Part model, mm, in its own coordinate system. A direction names the side the tool comes from. Round coordinates to 2 decimals unless told otherwise and drop trailing zeros. Write each loop counter-clockwise with the first axis right and the second up, starting at its lowest first coordinate (ties: lowest second). Pieces come first, ordered by that corner, then holes.
1) Saw through at A-A on y = -39.76. Write the cut outline in (x, z), and give its area (3 significant figures).
2) Which spindle directions (+Z, -Z, +X, -X, +Y, -Y) get a long thin tool onto all of the face, cutting with end or side? Do faces 1 (the flat face through (4, -15, 20)), 2 (the flat face through (4, 35.76, -16)), 3 (the cylindrical face through (2, 52, 0)). Say none if no direction does.
3) Saw through at D-D on z = -18.5. Write the cut outline in (x, y), and give its area (3 significant figures).
4) Saw through at C-C on y = 41.76. Write the cut outline in (x, z) (3 decimals).
5) Flat gauge pins, fed straight in: pin 1 (2.5 mm diameter, centred on x = 7, y = 51.5, fed in from +Z); pin 2 (1.5 mm diameter, centred on x = 5.5, y = 6.5, fed in from -Z); pin 3 (2.5 mm diameter, centred on x = 6.5, y = 52, fed in from -Z); pin 4 (5.5 mm diameter, centred on y = -39.76, z = 17, fed in from -X). Where does each tip first touch, or does it go through?
6) Drill centre lines: L1, parallel to Y at x = 2.5, z = 16; L2, parallel to Y at x = 4, z = 17; L3, parallel to Z at x = 4, y = 48. Where is each one in solid material? Low to high.
7) Pull direction Y, two halves, no side cores. Call faces 4 (the flat face through (7, 52, 1.25)), 5 (the flat face through (4, -47.76, 17)), 6 (the cylindrical face through (3.94, 38.83, 16.35)): +Y half, -Y half, draft (parallel to the pull), parting line (faces both ways), or undercut.
8) Saw through at B-B on x = 4. Count the separate pieces of the cut face and the enclosed holes in it, and give its area (3 significant figures).
```python
from build123d import *

# Parameters (mm, degrees)
SKETCH1_W                       = 46
SKETCH1_H                       = 95.52
BOSS_EXTRUDE1_DEPTH             = 8
F_6_0MM_CLEARANCE_DOWEL_HOLE1_D = 6
SKETCH4_W                       = 8
SKETCH4_H                       = 46
BOSS_EXTRUDE2_DEPTH             = 12
FILLET1_R                       = 10
SKETCH6_R                       = 2
CUT_EXTRUDE2_DEPTH              = 15
SKETCH9_W                       = 26
SKETCH9_H                       = 30.52
CUT_EXTRUDE5_DEPTH              = 65.531059189
F_6_0MM_CLEARANCE_DOWEL_HOLE2_D = 6
CUT_EXTRUDE13_DEPTH             = 65.531059189
SKETCH7_W                       = 2.5
SKETCH7_H                       = 15
CUT_EXTRUDE12_DEPTH             = 4
SKETCH16_W                      = 34
SKETCH16_H                      = 53
CUT_EXTRUDE9_DEPTH              = 65.531059294
CUT_EXTRUDE14_DEPTH             = 65.531059294
CUT_EXTRUDE15_DEPTH             = 65.531059294
FILLET2_START                   = -1
FILLET2_DEPTH                   = 10
SKETCH22_R                      = 3
CUT_EXTRUDE16_DEPTH             = 65.531059329


with BuildPart() as part:
    # Sketch1 → Boss-Extrude1 (new body)
    with BuildSketch(Plane(origin=(0, 0, 0), x_dir=(0, 0, -1), z_dir=(1, 0, 0))):
        Rectangle(SKETCH1_W, SKETCH1_H)
    extrude(amount=BOSS_EXTRUDE1_DEPTH)

    # Ø6.0mm Clearance Dowel Hole1 (through all)
    with Locations(Plane(origin=(8, 0, 0), x_dir=(0, 0, -1), z_dir=(1, 0, 0))):
        with Locations((-17, 41.76), (17, 41.76)):
            Hole(F_6_0MM_CLEARANCE_DOWEL_HOLE1_D / 2)

    # Sketch4 → Boss-Extrude2 (add)
    with BuildSketch(Plane(origin=(0, 47.76, 0), x_dir=(1, 0, 0), z_dir=(0, 1, 0))):
        with Locations((4, 0)):
            Rectangle(SKETCH4_W, SKETCH4_H)
    extrude(amount=BOSS_EXTRUDE2_DEPTH)

    # Fillet1
    fillet1_edges = [part.edges().sort_by_distance(p)[0] for p in [
        (4, 59.76, 23),
        (4, 59.76, -23),
    ]]
    fillet(fillet1_edges, radius=FILLET1_R)

    # Sketch6 → Cut-Extrude2 (cut)
    with BuildSketch(Plane(origin=(0, 59.76, 0), x_dir=(1, 0, 0), z_dir=(0, 1, 0))):
        with Locations(Location((4, 0, 0), (0, 0, 270))):
            Circle(SKETCH6_R)
    extrude(amount=-CUT_EXTRUDE2_DEPTH, mode=Mode.SUBTRACT)

    # Sketch9 → Cut-Extrude5 (cut, through all)
    with BuildSketch(Plane(origin=(8, 0, 0), x_dir=(0, 0, -1), z_dir=(1, 0, 0))):
        with Locations((10, 20.5)):
            Rectangle(SKETCH9_W, SKETCH9_H)
    extrude(amount=-CUT_EXTRUDE5_DEPTH, mode=Mode.SUBTRACT)

    # Ø6.0mm Clearance Dowel Hole2 (through all)
    with Locations(Plane(origin=(8, 0, 0), x_dir=(0, 0, -1), z_dir=(1, 0, 0))):
        with Locations((-17, -39.76)):
            Hole(F_6_0MM_CLEARANCE_DOWEL_HOLE2_D / 2)

    # Sketch14 → Cut-Extrude13 (cut, through all)
    with BuildSketch(Plane(origin=(8, 0, 0), x_dir=(0, 0, -1), z_dir=(1, 0, 0))):
        with BuildLine():
            Line((5, 40.013359235), (5, 35.76))
            Line((5, 35.76), (-5, 35.76))
            Line((-5, 35.76), (-5, 40.013359235))
            ThreePointArc((-5, 40.013359235), (0, 45.013359235), (5, 40.013359235))
        make_face()
    extrude(amount=-CUT_EXTRUDE13_DEPTH, mode=Mode.SUBTRACT)

    # Sketch7 → Cut-Extrude12 (cut)
    with BuildSketch(Plane(origin=(8, 0, 0), x_dir=(0, 0, -1), z_dir=(1, 0, 0))):
        with Locations((0, 52.26)):
            Rectangle(SKETCH7_W, SKETCH7_H)
    extrude(amount=-CUT_EXTRUDE12_DEPTH, mode=Mode.SUBTRACT)

    # Sketch16 → Cut-Extrude9 (cut, through all)
    with BuildSketch(Plane(origin=(8, 0, 0), x_dir=(0, 0, -1), z_dir=(1, 0, 0))):
        with Locations((6, -21.26)):
            Rectangle(SKETCH16_W, SKETCH16_H)
    extrude(amount=-CUT_EXTRUDE9_DEPTH, mode=Mode.SUBTRACT)

    # Sketch19 → Cut-Extrude14 (cut, through all)
    with BuildSketch(Plane(origin=(8, 0, 0), x_dir=(0, 0, -1), z_dir=(1, 0, 0))):
        Polygon((-5, 35.76), (3.485281374, 27.274718626), (10.556349186, 34.345786438), (2.071067812, 42.831067812), align=None)
    extrude(amount=-CUT_EXTRUDE14_DEPTH, mode=Mode.SUBTRACT)

    # Sketch21 → Cut-Extrude15 (cut, through all)
    with BuildSketch(Plane(origin=(8, 0, 0), x_dir=(0, 0, -1), z_dir=(1, 0, 0))):
        Polygon((-3, 7.538097039), (-5.298097039, 5.24), (-3, 5.24), align=None)
    extrude(amount=-CUT_EXTRUDE15_DEPTH, mode=Mode.SUBTRACT)

    # Fillet2: read off the stored shape, not the designer's step
    # Fillet2 outline → Fillet2 (cut)
    with BuildSketch(Plane.YZ.offset(FILLET2_START)):
        with BuildLine():
            add(Edge.make_bspline(
                [(40.779548187, -4.94094672), (39.810996275, -5.091139348), (39.117941215, -5.784194408)],
                knots=[0, 0, 0, 1, 1, 1], degree=2))
            ThreePointArc((40.779548187, -4.94094672), (40.397589895, -4.98521482), (40.013359235, -5))
            Line((40.013359235, -5), (39.902135624, -5))
            Line((39.902135624, -5), (39.117941215, -5.784194408))
        make_face()
    extrude(amount=FILLET2_DEPTH, mode=Mode.SUBTRACT)

    # Fillet3
    # a fillet whose section is not a circle: 3 mm, written as the material it adds along each edge
    with BuildSketch(Plane(origin=(8, 35.76, 5), x_dir=(0, 1, 0), z_dir=(-1, 0, 0))) as fillet3_piece_1:
        with BuildLine():
            Bezier((1.242640687, 0), (0, 0), (-0.878679656, 0.878679656), weights=[1, 1, 1])
            Line((-0.878679656, 0.878679656), (0, 0))
            Line((0, 0), (1.242640687, 0))
        make_face()
    extrude(amount=8)

    # Sketch22 → Cut-Extrude16 (cut, through all)
    with BuildSketch(Plane(origin=(8, 0, 0), x_dir=(0, 0, -1), z_dir=(1, 0, 0))):
        with Locations((-17, 0.39)):
            Circle(SKETCH22_R)
        with BuildLine():
            Line((-14, -9.77), (-14, -19.77))
            ThreePointArc((-14, -19.77), (-17, -22.77), (-20, -19.77))
            Line((-20, -19.77), (-20, -9.77))
            ThreePointArc((-20, -9.77), (-17, -6.77), (-14, -9.77))
        make_face()
    extrude(amount=-CUT_EXTRUDE16_DEPTH, mode=Mode.SUBTRACT)


solid = part.part
```
Completed:
1. outline: (0, 11) - (8, 11) - (8, 14) - (0, 14) - close; (0, 20) - (8, 20) - (8, 23) - (0, 23) - close
1. area: 48.0 mm2
2. face 1: +X, -X
2. face 2: -Z, +X, -X, -Y
2. face 3: +Y
3. outline: (0, 35.76) - (8, 35.76) - (8, 39.16) - (0, 39.16) - close; (0, 44.36) - (8, 44.36) - (8, 58.11) - (0, 58.11) - close
3. area: 137 mm2
4. outline: (0, -23) - (8, -23) - (8, -20) - (0, -20) - close; (0, -14) - (8, -14) - (8, -4.685) - (0, -4.685) - close; (0, 4.685) - (8, 4.685) - (8, 14) - (0, 14) - close; (0, 20) - (8, 20) - (8, 23) - (0, 23) - close
5. pin 1: stops at z = 22.99
5. pin 2: stops at z = 3.29
5. pin 3: stops at z = -22.95
5. pin 4: passes through
6. L1: y = -47.76 to -42.59, -36.93 to -22.6, -6.94 to -2.44, 3.22 to 38.93, 44.59 to 59.3
6. L2: y = -47.76 to -42.76, -36.76 to -22.77, -6.77 to -2.61, 3.39 to 38.76, 44.76 to 58.93
6. L3: z = -23 to -2, 2 to 23
7. face 4: draft
7. face 5: -Y half
7. face 6: undercut
8. separate pieces: 2
8. enclosed holes: 5
8. area: 1,950 mm2
